The model under review builds one solid part; all positions refer to its coordinate system, in mm. Face numbers are marked on the shaded views. A direction names the side the tool comes from. Coordinates: 2 decimals unless noted, no trailing zeros. Loops run counter-clockwise (first coordinate to the right, second up) from the corner with the lowest first, then second, coordinate; pieces in that order, holes last. Notation, with made-up numbers: M -33.5,79.5 L 22.5,79.5 A20 cw 22.5,85.5 Z; hole C 39.5,74 d4. An arc over 180 degrees is marked long. Use CSV: the item, a comma, the result in double quotes. Start each with the question number.
1. Draft analysis for pull direction X (two halves, no side actions). For the marked faces 4, 5 and 6, state which applies: +X half, -X half, draft (parallel to the pull), parting line (faces both ways), or undercut.
2. Tool access review of the marked faces 1, 2 and 3: name each direction out of +Z, -Z, +X, -X, +Y, -Y from which nothing blocks a thin tool from reaching the whole face with its end or side.
3. Add section D-D, the plane z = 10.5. Write out the cut boundary in (x, y).
4. Add section B-B, the plane y = -4.5. Write out the cut boundary in (x, z), then the cut area to 3 significant figures.
5. Add section A-A, the plane z = 12.75. Write out the cut boundary in (x, y), then the cut area to 3 significant figures.
6. Add section C-C, the plane x = 0. Write out the cut boundary in (y, z).
7. Clearance check with flat-ended pins moving along their axes: P1, Ø2, axis at x = -3.5, z = 7.5, coming from the +Y side; P2, Ø3.5, axis at x = -17.75, y = -1.62, coming from the -Z side; P3, Ø3.5, axis at x = -16.5, z = 1, coming from the -Y side; P4, Ø3, axis at x = -15.5, z = 7, coming from the -Y side. State where each tip first meets the part, or that it passes through.
8. For L1, parallel to Z at x = 19.5, y = 1; L2, parallel to Y at x = -15, z = 13.65; L3, parallel to X at y = 0.5, z = 6.5, list the stretches that pass through material, from the lowest coordinate up.
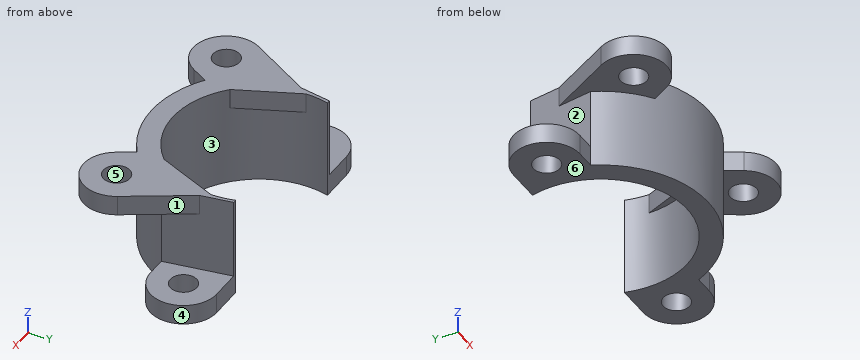
from build123d import *

# Parameters (mm, degrees)
ESBO_O1_R                = 2
RESSALTO_EXTRUS_O1_DEPTH = 3
RESSALTO_EXTRUS_O2_DEPTH = 12
ESBO_O3_R                = 2
RESSALTO_EXTRUS_O3_DEPTH = 3


with BuildPart() as part:
    # Esboço1 → Ressalto-extrusão1 (new body)
    with BuildSketch(Plane.XY):
        with BuildLine():
            Line((-17.75, 3.382927425), (-13.099117311, 3.382927425))
            Line((-13.099117311, 3.382927425), (-12.552123407, 3.382927425))
            ThreePointArc((-12.552123407, 3.382927425), (0, -13), (12.552123407, 3.382927425))
            Line((12.552123407, 3.382927425), (13.099117311, 3.382927425))
            Line((13.099117311, 3.382927425), (17.75, 3.382927425))
            ThreePointArc((17.75, 3.382927425), (22.75, -1.617072575), (17.75, -6.617072575))
            Line((17.75, -6.617072575), (14.779561157, -6.617072575))
            ThreePointArc((14.779561157, -6.617072575), (0, -16.193241721), (-14.779561157, -6.617072575))
            Line((-14.779561157, -6.617072575), (-17.75, -6.617072575))
            ThreePointArc((-17.75, -6.617072575), (-22.75, -1.617072575), (-17.75, 3.382927425))
        make_face()
        with Locations((-17.75, -1.617072575)):
            Circle(ESBO_O1_R, mode=Mode.SUBTRACT)
        with Locations((17.75, -1.617072575)):
            Circle(ESBO_O1_R, mode=Mode.SUBTRACT)
    extrude(amount=RESSALTO_EXTRUS_O1_DEPTH)

    # Esboço2 → Ressalto-extrusão2 (add)
    with BuildSketch(Plane.XY.offset(3)):
        with BuildLine():
            Line((13.099117311, 3.382927425), (14.779561157, -6.617072575))
            ThreePointArc((14.779561157, -6.617072575), (0, -16.193241721), (-14.779561157, -6.617072575))
            Line((-14.779561157, -6.617072575), (-13.099117311, 3.382927425))
            Line((-13.099117311, 3.382927425), (-12.552123407, 3.382927425))
            ThreePointArc((-12.552123407, 3.382927425), (0, -13), (12.552123407, 3.382927425))
            Line((12.552123407, 3.382927425), (13.099117311, 3.382927425))
        make_face()
    extrude(amount=RESSALTO_EXTRUS_O2_DEPTH)

    # Esboço3 → Ressalto-extrusão3 (add)
    with BuildSketch(Plane.XY.offset(15)):
        with BuildLine():
            Line((13.077187708, 0.083527365), (8.154782397, -11.379785765))
            Line((8.154782397, -11.379785765), (10.671688275, -15.731898104))
            ThreePointArc((10.671688275, -15.731898104), (17.503141549, -17.55706828), (19.328311725, -10.725615007))
            Line((19.328311725, -10.725615007), (13.077187708, 0.083527365))
        make_face()
        with Locations((15, -13.228756555)):
            Circle(ESBO_O3_R, mode=Mode.SUBTRACT)
        with BuildLine():
            Line((-10.671688275, -15.731898104), (-8.154782397, -11.379785765))
            Line((-8.154782397, -11.379785765), (-13.077187708, 0.083527365))
            Line((-13.077187708, 0.083527365), (-19.328311725, -10.725615007))
            ThreePointArc((-19.328311725, -10.725615007), (-17.503141549, -17.55706828), (-10.671688275, -15.731898104))
        make_face()
        with Locations((-15, -13.228756555)):
            Circle(ESBO_O3_R, mode=Mode.SUBTRACT)
    extrude(amount=-RESSALTO_EXTRUS_O3_DEPTH)


solid = part.part
Computed:
1,face 4,"+X half"
1,face 5,"undercut"
1,face 6,"draft"
2,face 1,"+Z, +X, +Y"
2,face 2,"-X, +Y"
2,face 3,"-Z"
3,outline,"M -14.78,-6.62 A16.19 ccw 14.78,-6.62 L 13.1,3.38 L 12.55,3.38 A13 cw long -12.55,3.38 L -13.1,3.38 Z"
4,outline,"M -21.84,0 L -12.2,0 L -12.2,12 L -11.11,12 L -11.11,15 L -15.73,15 L -15.73,12 L -14.42,12 L -14.42,3 L -21.84,3 Z; M 11.11,12 L 12.2,12 L 12.2,0 L 21.84,0 L 21.84,3 L 14.42,3 L 14.42,12 L 15.73,12 L 15.73,15 L 11.11,15 Z"
4,area,"126 mm^2"
5,outline,"M -19.33,-10.73 A5 ccw -10.67,-15.73 L -9.26,-13.29 A16.19 ccw 9.26,-13.29 L 10.67,-15.73 A5 ccw 19.33,-10.73 L 13.89,-1.32 L 13.1,3.38 L 12.55,3.38 A13 cw 13,-0.1 L 9.02,-9.36 A13 cw -9.02,-9.36 L -13,-0.1 A13 cw -12.55,3.38 L -13.1,3.38 L -13.89,-1.32 Z; hole C -15,-13.23 d4; hole C 15,-13.23 d4"
5,area,"292 mm^2"
6,outline,"M -16.19,0 L -13,0 L -13,15 L -16.19,15 Z"
7,P1,"stops at y = -12.2"
7,P2,"passes through"
7,P3,"stops at y = -6.68"
7,P4,"stops at y = -8.14"
8,L1,"z = 0 to 3"
8,L2,"y = -18.23 to -15.23, -11.23 to -3.24"
8,L3,"x = -13.58 to -12.99, 12.99 to 13.58"
